Here's how the part is built. I have some questions about the finished solid (model axes, mm). Round coordinates to 2 decimals unless told otherwise and drop trailing zeros. Write each loop counter-clockwise with the first axis right and the second up, starting at its lowest first coordinate (ties: lowest second). Pieces come first, ordered by that corner, then holes. Notation, with made-up numbers: (54, 61) - (94, 61) arc R14 ccw to (94, 79) - close; hole circle Ø3 at (-8, 47.25). An arc over 180 degrees is marked (long way). Write item = value, one per line. Start each with the question number.
Item 1: Thinking about a two-plate mould opening in Z: for faces 1 (the face through (0, 2, 0)), 2 (the face through (0, 0, 0)), which applies, pulls with the +Z half, pulls with the -Z half, needs draft (parallel to the pull), parting line crosses it, or undercut?
Item 2: If I drill on line 1 along Z through (x, y) = (17.5, 9.5); line 2 along Z through (x, y) = (18, 2.25); line 3 along Z through (x, y) = (20, 1.5), over which ranges is the centre line in solid material (lowest first)? Write a range as [from, to].
Item 3: If we section it at A-A (y = 7.75): Please give me the cut outline in (x, z).
Item 4: For P1, Ø2, axis at x = 20, y = 5.5, coming from the -Z side; P2, Ø4, axis at y = 3, z = -2, coming from the +X side; P3, Ø1, axis at x = -4, z = 0, coming from the +Y side, each with a flat end and sliding along its axis, tell me the tip position at first contact or that it passes through.
Item 5: If we section it at C-C (y = 2.75): Please give me the cut outline in (x, z), and give its area (3 significant figures).
```python
from build123d import *

# Parameters (mm, degrees)
BOSS_EXTRUDE1_DEPTH = 27.5
CUT_EXTRUDE1_DEPTH  = 56
FILLET1_R           = 0.466499
FILLET2_R           = 0.466369
FILLET3_R           = 0.466369
FILLET4_R           = 0.466499
FILLET5_R           = 0.4


with BuildPart() as part:
    # Sketch1 → Boss-Extrude1 (new body, symmetric)
    with BuildSketch(Plane(origin=(0, 0, 0), x_dir=(0, 0, -1), z_dir=(1, 0, 0))):
        Polygon((-4.15, 11.25), (-4.25, 0), (4.25, 0), (4.15, 11.25), align=None)
    extrude(amount=BOSS_EXTRUDE1_DEPTH, both=True)

    # Sketch2 → Cut-Extrude1 (cut, through all)
    with BuildSketch(Plane(origin=(27.5, 0, 0), x_dir=(0, 0, -1), z_dir=(1, 0, 0))):
        with BuildLine():
            Line((-0.8, 11.25), (-0.725, 2.247917221))
            ThreePointArc((-0.725, 2.247917221), (-0.651047458, 2.072488458), (-0.475008676, 2))
            Line((-0.475008676, 2), (0.475008676, 2))
            ThreePointArc((0.475008676, 2), (0.651047458, 2.072488458), (0.725, 2.247917221))
            Line((0.725, 2.247917221), (0.8, 11.25))
            Line((0.8, 11.25), (-0.8, 11.25))
        make_face()
        with BuildLine():
            Line((-3.225, 11.25), (-1.725, 11.25))
            Line((-1.725, 11.25), (-1.8, 2.247917221))
            ThreePointArc((-1.8, 2.247917221), (-1.873952542, 2.072488458), (-2.049991324, 2))
            Line((-2.049991324, 2), (-2.900008676, 2))
            ThreePointArc((-2.900008676, 2), (-3.076047458, 2.072488458), (-3.15, 2.247917221))
            Line((-3.15, 2.247917221), (-3.225, 11.25))
        make_face()
        with BuildLine():
            Line((3.225, 11.25), (1.725, 11.25))
            Line((1.725, 11.25), (1.8, 2.247917221))
            ThreePointArc((1.8, 2.247917221), (1.873952542, 2.072488458), (2.049991324, 2))
            Line((2.049991324, 2), (2.900008676, 2))
            ThreePointArc((2.900008676, 2), (3.076047458, 2.072488458), (3.15, 2.247917221))
            Line((3.15, 2.247917221), (3.225, 11.25))
        make_face()
    extrude(amount=-CUT_EXTRUDE1_DEPTH, mode=Mode.SUBTRACT)

    # Fillet1
    fillet1_edges = [part.edges().sort_by_distance(p)[0] for p in [
        (0, 11.25, 3.225),
        (0, 11.25, 4.15),
    ]]
    fillet(fillet1_edges, radius=FILLET1_R)

    # Fillet2
    fillet2_edges = [part.edges().sort_by_distance(p)[0] for p in [
        (0, 11.25, 0.8),
        (0, 11.25, 1.725),
    ]]
    fillet(fillet2_edges, radius=FILLET2_R)

    # Fillet3
    fillet3_edges = [part.edges().sort_by_distance(p)[0] for p in [
        (0, 11.25, -0.8),
        (0, 11.25, -1.725),
    ]]
    fillet(fillet3_edges, radius=FILLET3_R)

    # Fillet4
    fillet4_edges = [part.edges().sort_by_distance(p)[0] for p in [
        (0, 11.25, -3.225),
        (0, 11.25, -4.15),
    ]]
    fillet(fillet4_edges, radius=FILLET4_R)

    # Fillet5
    fillet5_edges = [part.edges().sort_by_distance(p)[0] for p in [
        (0, 0, -4.25),
        (0, 0, 4.25),
    ]]
    fillet(fillet5_edges, radius=FILLET5_R)


solid = part.part
```
Reply:
q1.face_1 = undercut
q1.face_2 = needs draft
q2.line_1 = [-4.17, -3.21], [-1.74, -0.79], [0.79, 1.74], [3.21, 4.17]
q2.line_2 = [-4.23, -3.15], [-1.8, -0.73], [0.73, 1.8], [3.15, 4.23]
q2.line_3 = [-4.24, 4.24]
q3.outline = (-27.5, -4.18) - (27.5, -4.18) - (27.5, -3.2) - (-27.5, -3.2) - close; (-27.5, -1.75) - (27.5, -1.75) - (27.5, -0.77) - (-27.5, -0.77) - close; (-27.5, 0.77) - (27.5, 0.77) - (27.5, 1.75) - (-27.5, 1.75) - close; (-27.5, 3.2) - (27.5, 3.2) - (27.5, 4.18) - (-27.5, 4.18) - close
q4.P1 = -4.21
q4.P2 = 27.5
q4.P3 = 2
q5.outline = (-27.5, -4.23) - (27.5, -4.23) - (27.5, -3.15) - (-27.5, -3.15) - close; (-27.5, -1.8) - (27.5, -1.8) - (27.5, -0.73) - (-27.5, -0.73) - close; (-27.5, 0.73) - (27.5, 0.73) - (27.5, 1.8) - (-27.5, 1.8) - close; (-27.5, 3.15) - (27.5, 3.15) - (27.5, 4.23) - (-27.5, 4.23) - close
q5.area = 235 mm2
